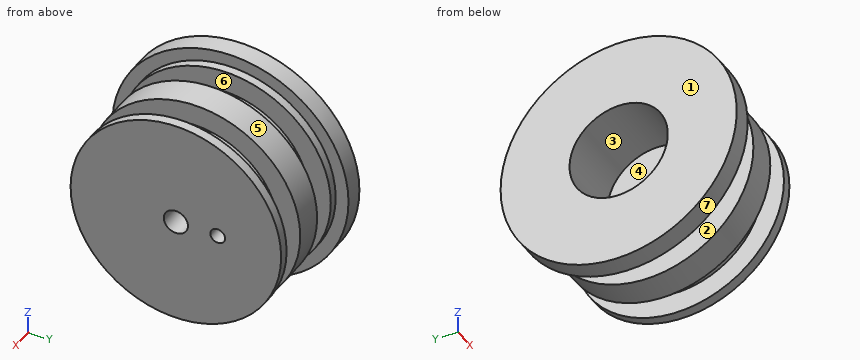
Autodesk Inventor part; units mm, degrees
ref_plane "YZ Plane" through (0, 0, 0) normal (1, 0, 0) x (0, 1, 0)
ref_plane "XZ Plane" through (0, 0, 0) normal (0, 1, 0) x (-1, 0, 0)
ref_plane "XY Plane" through (0, 0, 0) normal (0, 0, 1) x (1, 0, 0)
sketch "Skizze1" plane through (0, 0, 0) normal (0, 0, 1) x (1, 0, 0)
  line L0 (-2.4, 0) -> (14.4, 0)
  line L1 (0, -2.4) -> (0, 14.4)
  line L2 (0, 5) -> (7, 5)
  line L3 (7, 5) -> (7, 0)
  line L4 (7, 0) -> (12, 0)
  line L5 (12, 0) -> (12, 10.7)
  line L6 (12, 10.7) -> (11, 10.7)
  line L7 (11, 10.7) -> (11, 8.5)
  line L8 (11, 8.5) -> (8.5, 8.5)
  line L9 (8.5, 8.5) -> (8.5, 10.7)
  line L10 (8.5, 10.7) -> (5.4, 10.7)
  line L11 (5.4, 10.7) -> (5.4, 8.5)
  line L12 (5.4, 8.5) -> (2.9, 8.5)
  line L13 (2.9, 8.5) -> (2.9, 10.7)
  line L14 (2.9, 10.7) -> (2, 10.7)
  line L15 (2, 10.7) -> (2, 12)
  line L16 (2, 12) -> (0, 12)
  line L17 (0, 12) -> (0, 5)
  point P0 (0, 0)
  dimension "d0" = 24
  dimension "d1" = 10
  dimension "d2" = 17
  dimension "d3" = 21.4
  dimension "d4" = 2.5
  dimension "d5" = 2.5
  dimension "d7" = 1
  dimension "d8" = 6.6
  dimension "d9" = 12
  dimension "d11" = 10
  dimension "d12" = 7
revolve "Umdrehung1" add sketch "Skizze1" angle 360 about axis through (-10, 0, 0) along (1, 0, 0) contours L3 L2 L1 L16 L15 L14 L13 L12 L11 L10 L9 L8 L7 L6 L5 L0
sketch "Skizze2" plane through (7, 0, 0) normal (-1, 0, 0) x (0, 0, 1)
  point P0 (0, 0)
  point P1 (0, 0)
hole "Bohrung1" at (7, 0, 0) direction (1, 0, 0) diameter 2.459 end through all countersink diameter 3.5 countersink angle 90
sketch "Skizze3" plane through (7, 0, 0) normal (-1, 0, 0) x (0, 0, 1)
  line L0 (-16.8, 0) -> (16.8, 0)
  line L1 (0, -16.8) -> (0, 16.8)
  circle A0 centre (0, 0) radius 5
  point P0 (0, 4.25)
  dimension "d21" = 4.25
hole "Bohrung2" at (7, 4.25, 0) direction (1, 0, 0) diameter 1.5 end through all
properties part number "Innenflansch"
Part model, mm, in its own coordinate system. Face numbers are marked on the shaded views. A direction names the side the tool comes from. Give positions to 0.01 mm unless a question says otherwise; leave off trailing zeros. Write each loop counter-clockwise with the first axis right and the second up, starting at its lowest first coordinate (ties: lowest second). Pieces come first, ordered by that corner, then holes. Notation, with made-up numbers: M 22.25,68.25 L 73.25,68.25 A17 ccw 73.25,77.25 Z; hole C -13.5,29.5 d2. An arc over 180 degrees is marked long. Use CSV: the item, a comma, the result in double quotes.
Item 1: Slice it at D-D on y = 7.5. Write the cut outline in (x, z).
Taken from the geometry:
outline,"M 0,-9.37 L 2,-9.37 L 2,-7.63 L 2.9,-7.63 L 2.9,-4 L 5.4,-4 L 5.4,-7.63 L 8.5,-7.63 L 8.5,-4 L 11,-4 L 11,-7.63 L 12,-7.63 L 12,7.63 L 11,7.63 L 11,4 L 8.5,4 L 8.5,7.63 L 5.4,7.63 L 5.4,4 L 2.9,4 L 2.9,7.63 L 2,7.63 L 2,9.37 L 0,9.37 Z"
Item 2: Slice it at B-B on x = 4.75. Write the cut outline in (y, z).
Taken from the geometry:
outline,"C 0,0 d17; hole C 0,0 d10"
Item 3: Pin check, flat tips, straight feed: P1, Ø6, axis at y = 0, z = 0, coming from the -X side; P2, Ø4, axis at x = 7.5, y = -3.5, coming from the -Z side; P3, Ø3, axis at x = 2, z = -3, coming from the +Y side. Stop position of each tip, or through.
Taken from the geometry:
P1,"stops at x = 7"
P2,"stops at z = -10.59"
P3,"stops at y = 11.91"
Item 4: Slice it at C-C on z = 10.25. Write the cut outline in (x, y).
Taken from the geometry:
outline,"M 0,-6.24 L 2,-6.24 L 2,-3.07 L 2.9,-3.07 L 2.9,3.07 L 2,3.07 L 2,6.24 L 0,6.24 Z; M 5.4,-3.07 L 8.5,-3.07 L 8.5,3.07 L 5.4,3.07 Z; M 11,-3.07 L 12,-3.07 L 12,3.07 L 11,3.07 Z"
Item 5: Drill centre lines: probe 1 along X at (y, z) = (-7, -7.25); probe 2 along Z at (x, y) = (4.5, 0); probe 3 along Z at (x, y) = (8.8, 0). Where is each one in solid material? Low to high.
Taken from the geometry:
probe 1,"x = 0 to 2.9, 5.4 to 8.5, 11 to 12"
probe 2,"z = -8.5 to -5, 5 to 8.5"
probe 3,"z = -8.5 to -1.23, 1.23 to 8.5"
Item 6: Pull direction X, two halves, no side cores. Call the marked faces 1, 2 and 3: +X half, -X half, draft (parallel to the pull), parting line (faces both ways), or undercut.
Taken from the geometry:
face 1,"-X half"
face 2,"undercut"
face 3,"draft"
Item 7: Which spindle directions (+Z, -Z, +X, -X, +Y, -Y) get a long thin tool onto all of the face, cutting with end or side? Do the marked faces 4, 5, 6 and 7. Say none if no direction does.
Taken from the geometry:
face 4,"-X"
face 5,"+X"
face 6,"none"
face 7,"+X, -X"
